Verification items for the finished model (mm, model axes). A direction names the side the tool comes from. Round coordinates to 2 decimals unless told otherwise and drop trailing zeros. Loops run counter-clockwise (first coordinate to the right, second up) from the corner with the lowest first, then second, coordinate; pieces in that order, holes last. Notation, with made-up numbers: (54, 4) - (95, 4) arc R19 ccw to (95, 32) - close; hole circle Ø5 at (28, -29.5). An arc over 180 degrees is marked (long way). Use CSV: the item, a comma, the result in double quotes.
```python
from build123d import *

# Parameters (mm, degrees)
BOSS_EXTRUDE2_DEPTH = 16
SKETCH7_R           = 2.25
CUT_EXTRUDE4_DEPTH  = 30.201645329
SKETCH6_R           = 1.25
SKETCH6_W           = 8
SKETCH6_H           = 20
CUT_EXTRUDE5_DEPTH  = 28.734295303
FILLET2_R           = 1


with BuildPart() as part:
    # Sketch2 → Boss-Extrude2 (new body)
    with BuildSketch(Plane.XY):
        with BuildLine():
            Line((-2.157979857, -1.939692621), (-11.554906065, -5.359894054))
            Line((-11.554906065, -5.359894054), (-10.528845635, -8.178971916))
            Line((-10.528845635, -8.178971916), (-1.131919427, -4.758770483))
            ThreePointArc((-1.131919427, -4.758770483), (0.776608177, -3.294305745), (1.5, -1))
            Line((1.5, -1), (1.5, 20.3))
            Line((1.5, 20.3), (-1.5, 20.3))
            Line((-1.5, 20.3), (-1.5, -1))
            ThreePointArc((-1.5, -1), (-1.680847956, -1.573576436), (-2.157979857, -1.939692621))
        make_face()
    extrude(amount=-BOSS_EXTRUDE2_DEPTH)

    # Sketch7 → Cut-Extrude4 (cut, through all)
    with BuildSketch(Plane(origin=(0.370969502, -1.01923033, 0), x_dir=(0.9396926207859104, 0.34202014332566305, 0), z_dir=(-0.3420201433256631, 0.9396926207859105, 0))):
        with Locations(Location((-7.691251695, 11, 0), (0, 0, 180))):
            Circle(SKETCH7_R)
    extrude(amount=-CUT_EXTRUDE4_DEPTH, mode=Mode.SUBTRACT)

    # Sketch6 → Cut-Extrude5 (cut, through all)
    with BuildSketch(Plane.ZY.offset(1.5)):
        with Locations(Location((-4, 17.8, 0), (0, 0, 270))):
            Circle(SKETCH6_R)
        with Locations(Location((-4, 1.5, 0), (0, 0, 270))):
            Circle(SKETCH6_R)
        with Locations((-12, 10.3)):
            Rectangle(SKETCH6_W, SKETCH6_H)
    extrude(amount=-CUT_EXTRUDE5_DEPTH, mode=Mode.SUBTRACT)

    # Fillet2
    fillet2_edges = [part.edges().sort_by_distance(p)[0] for p in [
        (0, 0.3, -16),
        (0, 20.3, -8),
        (0, 0.3, -8),
    ]]
    fillet(fillet2_edges, radius=FILLET2_R)


solid = part.part
```
1) Cross-section at A-A, the plane z = -4. Record the cut outline in (x, y).
Returned:
outline,"(-11.55, -5.36) - (-10.53, -8.18) - (-1.13, -4.76) arc R4 ccw to (1.5, -1) - (1.5, 0.25) - (-1.5, 0.25) - (-1.5, -1) arc R1 cw to (-2.16, -1.94) - close; (-1.5, 2.75) - (1.5, 2.75) - (1.5, 16.55) - (-1.5, 16.55) - close; (-1.5, 19.05) - (1.5, 19.05) - (1.5, 20.3) - (-1.5, 20.3) - close"
2) Cross-section at D-D, the plane x = -0.75. Record the cut outline in (y, z), then the cut area to 3 significant figures.
Returned:
outline,"(-4.6, -16) - (-0.7, -16) arc R1 ccw to (0.3, -15) - (0.3, -9) arc R1 cw to (1.3, -8) - (19.3, -8) arc R1 ccw to (20.3, -7) - (20.3, 0) - (-4.6, 0) - close; hole circle Ø2.5 at (1.5, -4); hole circle Ø2.5 at (17.8, -4)"
area,"228 mm²"
3) Thickness scan on probe 1 along Z at (x, y) = (0.6, 17.8); probe 2 along X at (y, z) = (-0.25, -10.25); probe 3 along Z at (x, y) = (0, 3). Record the ranges inside material, lowest first. Write a range as [from, to].
Returned:
probe 1,"z = [-8, -5.25], [-2.75, 0]"
probe 2,"x = [-1.5, 1.5]"
probe 3,"z = [-8, 0]"
4) Access from +Z, -Z, +X, -X, +Y, -Y to the whole of each face (thin tool, end or side, straight path). Record for faces 1 (the face through (-0.021, 0.923, -5.109)), 2 (the face through (-1.5, 10, -4)), 3 (the face through (0, 10, -8)).
Returned:
face 1,"+X, -X"
face 2,"+Z, -Z, -X, +Y"
face 3,"-Z, +X, -X, +Y"
5) Cross-section at C-C, the plane z = -6.5. Record the cut outline in (x, y).
Returned:
outline,"(-11.55, -5.36) - (-10.53, -8.18) - (-1.13, -4.76) arc R4 ccw to (1.5, -1) - (1.5, 20.3) - (-1.5, 20.3) - (-1.5, -1) arc R1 cw to (-2.16, -1.94) - close"
6) Cross-section at B-B, the plane y = 17.8. Record the cut outline in (x, z), then the cut area to 3 significant figures.
Returned:
outline,"(-1.5, -8) - (1.5, -8) - (1.5, -5.25) - (-1.5, -5.25) - close; (-1.5, -2.75) - (1.5, -2.75) - (1.5, 0) - (-1.5, 0) - close"
area,"16.5 mm²"
7) Gauge pin test, flat ends, axial feed: pin 1 Ø1 at (x, y) = (-1, 0) entering from -Z; pin 2 Ø3 at (y, z) = (12.5, -4.5) entering from -X; pin 3 Ø0.9 at (x, y) = (-0.5, 9) entering from -Z. Record the tip position at first contact, or that the pin passes through.
Returned:
pin 1,"stops at z = -15.98"
pin 2,"stops at x = -1.5"
pin 3,"stops at z = -8"
8) Mould release check, pull along Z, two halves, no side actions. Record for faces 4 (the face through (-6.08, -4.94, -8.77)), 5 (the face through (-1, 4, 0)), 6 (the face through (0.76, -3.32, -7.89)), 7 (the face through (0.021, 0.585, -8.301)): +Z half, -Z half, draft (parallel to the pull), parting line (faces both ways), or undercut.
Returned:
face 4,"undercut"
face 5,"+Z half"
face 6,"draft"
face 7,"-Z half"
